```python
from build123d import *

# Parameters (mm, degrees)
BOSS_EXTRUDE1_DEPTH = 20
SKETCH3_R           = 2.1
CUT_EXTRUDE2_DEPTH  = 30
SKETCH4_R           = 8.25
CUT_EXTRUDE3_DEPTH  = 5
FILLET1_R           = 1
FILLET2_R           = 1
FILLET3_R           = 1
SKETCH5_R           = 2.75
CUT_EXTRUDE4_DEPTH  = 20
SKETCH6_R           = 5
CUT_EXTRUDE5_DEPTH  = 4


with BuildPart() as part:
    # Sketch1 → Boss-Extrude1 (new body)
    with BuildSketch(Plane(origin=(0, 0, 0), x_dir=(1, 0, 0), z_dir=(0, 1, 0))):
        with BuildLine():
            Line((0, 44.25), (0, 75))
            ThreePointArc((0, 75), (75, 0), (0, -75))
            Line((0, -75), (0, -44.25))
            ThreePointArc((0, -44.25), (44.25, 0), (0, 44.25))
        make_face()
    extrude(amount=BOSS_EXTRUDE1_DEPTH)

    # Sketch3 → Cut-Extrude2 (cut)
    with BuildSketch(Plane.ZY):
        with Locations((-63, 10)):
            Circle(SKETCH3_R)
        with Locations((63, 10)):
            Circle(SKETCH3_R)
    extrude(amount=-CUT_EXTRUDE2_DEPTH, mode=Mode.SUBTRACT)

    # Sketch4 → Cut-Extrude3 (cut)
    with BuildSketch(Plane(origin=(0, 20, 0), x_dir=(1, 0, 0), z_dir=(0, 1, 0))):
        with Locations(Location((61.63, 0, 0), (0, 0, 270))):
            Circle(SKETCH4_R)
    extrude(amount=-CUT_EXTRUDE3_DEPTH, mode=Mode.SUBTRACT)

    # Fillet1
    fillet1_edges = [part.edges().sort_by_distance(p)[0] for p in [
        (61.63, 20, -8.25),
    ]]
    fillet(fillet1_edges, radius=FILLET1_R)

    # Fillet2
    fillet2_edges = [part.edges().sort_by_distance(p)[0] for p in [
        (44.25, 20, 0),
    ]]
    fillet(fillet2_edges, radius=FILLET2_R)

    # Fillet3
    # the kernel refuses this fillet: 1 mm, written as the material it takes off along each edge
    with BuildSketch(Plane(origin=(0, 20, -42.75), x_dir=(1, 0, 0), z_dir=(0, 0, -1)), Plane(origin=(0, 20, 77.5), x_dir=(1, 0, 0), z_dir=(0, 0, -1))) as fillet3_piece_1:
        with BuildLine():
            CenterArc((FILLET3_R, FILLET3_R), FILLET3_R, 180, 90)
            Line((0, FILLET3_R), (0, 0))
            Line((0, 0), (FILLET3_R, 0))
        make_face()
    extrude(amount=34.75, mode=Mode.SUBTRACT)
    with BuildSketch(Plane(origin=(0, 20, 0), x_dir=(-0.033380737313120155, 0, -0.9994427079009744), z_dir=(-0.9994427079009744, 0, 0.033380737313120155))) as fillet3_piece_2:
        with BuildLine():
            CenterArc((75 - FILLET3_R, FILLET3_R), FILLET3_R, 270, 90)
            Line((75, FILLET3_R), (75, 0))
            Line((75, 0), (75 - FILLET3_R, 0))
        make_face()
    revolve(axis=Axis((0, 20, 0), (0, -1, 0)), revolution_arc=183.825861464, mode=Mode.SUBTRACT)

    # Sketch5 → Cut-Extrude4 (cut)
    with BuildSketch(Plane(origin=(0, 15, 0), x_dir=(1, 0, 0), z_dir=(0, 1, 0))):
        with Locations(Location((61.63, 0, 0), (0, 0, 270))):
            Circle(SKETCH5_R)
    extrude(amount=-CUT_EXTRUDE4_DEPTH, mode=Mode.SUBTRACT)

    # Sketch6 → Cut-Extrude5 (cut)
    with BuildSketch(Plane.XZ):
        with Locations(Location((61.63, 0, 0), (0, 0, 270))):
            Circle(SKETCH6_R)
    extrude(amount=-CUT_EXTRUDE5_DEPTH, mode=Mode.SUBTRACT)


solid = part.part
```
Input: part model. Units: mm. Frame: model coordinates. A direction names the side the tool comes from. Round coordinates to 2 decimals unless told otherwise and drop trailing zeros. One line per item, written item: value. Start each with the question number.
(1) Draft query along Y for faces 5 (the flat face through (46, 20, -1)), 6 (the cylindrical face through (74.98, 9.37, -1.65)), 7 (the flat face through (30, 10, -63)), 8 (the cylindrical face through (14.79, 10.631, -60.997)). Return one class per face: +Y half, -Y half, draft (parallel to the pull), parting line (faces both ways), or undercut.
(2) Contact query for flat-ended pins moving along their axis: P1, Ø1.5, axis at x = 37.5, y = 18, coming from the -Z side; P2, Ø10, axis at x = 61.63, z = 0, coming from the +Y side; P3, Ø5, axis at y = 10, z = -63, coming from the +X side. Output: stop coordinate, or through.
(3) Ray query, line 1 (Y direction, x = 18.5, z = -63); line 2 (X direction, y = 17.1, z = 0); line 3 (X direction, y = 8.5, z = 0). Return the intervals inside material, ascending. Write a range as [from, to].
(4) Section A-A, the plane x = 19.5. Count the separate pieces of the cut face and the enclosed holes in it, plus the area to 3 significant figures.
(5) Access query for faces 1 (the flat face through (0, 9, -59)), 2 (the flat face through (59, 4, -2)), 3 (the cylindrical face through (14.79, 10.631, 65.003)), 4 (the flat face through (64, 15, -2)). Directions: +Z, -Z, +X, -X, +Y, -Y. A direction counts if a zero-diameter tool reaches every point of the face in a straight line with its end or side. Return the directions, or none.
Results below:
1. face 5: +Y half
1. face 6: draft
1. face 7: undercut
1. face 8: undercut
2. P1: z = -65.38
2. P2: y = 15
2. P3: x = 44.33
3. line 1: [0, 7.9], [12.1, 20]
3. line 2: [44.25, 53.38], [69.88, 75]
3. line 3: [44.25, 58.88], [64.38, 75]
4. separate pieces: 2
4. enclosed holes: 2
4. area: 1,280 mm^2
5. face 1: +Z, -Z, -X, +Y, -Y
5. face 2: -Y
5. face 3: -X
5. face 4: +Y
